Source: CAD feature listing. Evaluate the final solid. Frame: model axes, mm. A direction names the side the tool comes from. Round coordinates to 2 decimals unless told otherwise and drop trailing zeros. Order: outer loops, then holes, each group sorted by start corner. A loop starts at its lowest first (then second) coordinate and runs counter-clockwise, first axis right, second up. Notation, with made-up numbers: (-24.75, 9.5) -> (19.25, 9.5) arc R15 cw to (19.25, 21.5) -> close; hole circle Ø5 at (23, -39.5). An arc over 180 degrees is marked (long way). Write item = value, one per line. Start each with the question number.
(1) Draft query along Z for faces 1 (the face through (12, 46, -65)), 2 (the face through (7.01, 51.357, -126.748)), 3 (the face through (6, 15, 0)), 4 (the face through (7, 33, -160)). Return one class per face: released by +Z, released by -Z, zero draft, split by the parting line, or undercut.
(2) Ray query, line 1 (Y direction, x = -5, z = -130); line 2 (Z direction, x = -30, y = 41.5); line 3 (X direction, y = 38, z = -84.5). Return the intervals inside material, ascending.
(3) Contact query for flat-ended pins moving along their axis: pin 1 Ø9.5 at (x, y) = (29, 45.5) entering from +Z; pin 2 Ø1 at (x, z) = (-4, -59.5) entering from +Y; pin 3 Ø12 at (x, y) = (43.5, 75) entering from +Z. Output: stop coordinate, or through.
(4) Cut plane D-D on z = -110.5. Return the cut outline in (x, y), then the cut area to 3 significant figures.
(5) Cut plane C-C on y = 71.5. Return the cut outline in (x, z), then the cut area to 3 significant figures.
(6) Cut plane B-B on x = -17.5. Return the cut outline in (y, z).
(7) Cut plane A-A on z = -130. Return the cut outline in (x, y).
(8) Reachability of faces 5 (the face through (-16, 24, -49)), 6 (the face through (44.478, 39, -109)), 7 (the face through (28, 45, -100)), 8 (the face through (6, 10, -79)), 9 (the face through (-37, 12, -79)) from +Z, -Z, +X, -X, +Y, -Y: full face, straight path, thin tool, end or side. Return the list, or none.
from build123d import *

# Parameters (mm, degrees)
BOSS_EXTRUDE1_DEPTH = 160
SKETCH2_R           = 15
BOSS_EXTRUDE2_DEPTH = 76
BOSS_EXTRUDE3_DEPTH = 12


with BuildPart() as part:
    # Sketch1 → Boss-Extrude1 (new body)
    with BuildSketch(Plane.XY):
        Polygon((-43.521594684, 12), (-43.521594684, 0), (-19.521594684, 0), (-19.521594684, 10), (32.478405316, 10), (32.478405316, 0), (56.478405316, 0), (56.478405316, 12), (44.478405316, 12), (44.478405316, 24), (-31.521594684, 24), (-31.521594684, 12), align=None)
    extrude(amount=-BOSS_EXTRUDE1_DEPTH)

    # Sketch2 → Boss-Extrude2 (add)
    with BuildSketch(Plane(origin=(44.478405316, 0, 0), x_dir=(0, 0, -1), z_dir=(1, 0, 0))):
        with BuildLine():
            Line((100, 24), (160, 24))
            Line((160, 24), (160, 66))
            ThreePointArc((160, 66), (130, 96), (100, 66))
            Line((100, 66), (100, 24))
        make_face()
        with Locations((130, 66)):
            Circle(SKETCH2_R, mode=Mode.SUBTRACT)
    extrude(amount=-BOSS_EXTRUDE2_DEPTH)

    # Sketch8 → Boss-Extrude3 (add)
    with BuildSketch(Plane(origin=(0, 0, 0), x_dir=(0, 0, -1), z_dir=(1, 0, 0))):
        Polygon((0, 24), (109.656121138, 86.535715549), (109.656121138, 24), align=None)
    extrude(amount=BOSS_EXTRUDE3_DEPTH)


solid = part.part
Evaluation:
q1.face_1 = zero draft
q1.face_2 = undercut
q1.face_3 = released by +Z
q1.face_4 = released by -Z
q2.line_1 = 10 to 51, 81 to 96
q2.line_2 = -160 to -100
q2.line_3 = 0 to 12
q3.pin_1 = -100
q3.pin_2 = 24
q3.pin_3 = -100.15
q4.outline = (-43.52, 0) -> (-19.52, 0) -> (-19.52, 10) -> (32.48, 10) -> (32.48, 0) -> (56.48, 0) -> (56.48, 12) -> (44.48, 12) -> (44.48, 88.8) -> (-31.52, 88.8) -> (-31.52, 12) -> (-43.52, 12) -> close
q4.area = 6,520 mm^2
q5.outline = (-31.52, -159.49) -> (44.48, -159.49) -> (44.48, -143.96) -> (-31.52, -143.96) -> close; (-31.52, -116.04) -> (44.48, -116.04) -> (44.48, -100.51) -> (12, -100.51) -> (12, -83.29) -> (0, -83.29) -> (0, -100.51) -> (-31.52, -100.51) -> close
q5.area = 2,570 mm^2
q6.outline = (10, -160) -> (66, -160) arc R30 ccw to (66, -100) -> (24, -100) -> (24, 0) -> (10, 0) -> close; hole circle Ø30 at (66, -130)
q7.outline = (-43.52, 0) -> (-19.52, 0) -> (-19.52, 10) -> (32.48, 10) -> (32.48, 0) -> (56.48, 0) -> (56.48, 12) -> (44.48, 12) -> (44.48, 51) -> (-31.52, 51) -> (-31.52, 12) -> (-43.52, 12) -> close; (-31.52, 81) -> (44.48, 81) -> (44.48, 96) -> (-31.52, 96) -> close
q8.face_5 = +Z, -X, +Y
q8.face_6 = +Z, -Z, +X, +Y
q8.face_7 = +Z, +X, +Y
q8.face_8 = +Z, -Z, -Y
q8.face_9 = +Z, -Z, -X, +Y
